Could you check a few things on this model? Use its own coordinates, in mm. A direction names the side the tool comes from. Coordinates: 2 decimals unless noted, no trailing zeros. Loops run counter-clockwise (first coordinate to the right, second up) from the corner with the lowest first, then second, coordinate; pieces in that order, holes last.
1) Imagine slicing it at A-A on z = 27.5. Please give me the cut outline in (x, y) (3 decimals).
2) Imagine slicing it at D-D on x = 36.5. Please give me the cut outline in (y, z), plus the area to 3 significant figures.
3) Imagine slicing it at C-C on z = 10. Please give me the cut outline in (x, y) (3 decimals), plus the area to 3 significant figures.
4) For faces 4 (the face through (67.07, -3, 11.686)), 5 (the face through (23.337, -4.217, 28.465)), 6 (the face through (36, -4, 26)), 7 (the face through (4.93, -5.15, 11.686)), which set-ups out of +Z, -Z, +X, -X, +Y, -Y let a thin tool reach every point of the face, with its end or its side?
5) If I drill on line 1 along Y through (x, z) = (50, 29); line 2 along X through (y, z) = (-3, 28.9); line 3 along Z through (x, y) = (66, -4), over which ranges is the centre line in solid material (lowest first)?
6) Will these pins go through, and if not, where does the flat tip stop? P1, Ø3.5, axis at y = -4.075, z = 10, coming from the +X side; P2, Ø1.5, axis at y = -6, z = 28.5, coming from the -X side; P3, Ø1.5, axis at y = -4, z = 21, coming from the +X side.
7) Thinking about a two-plate mould opening in Y: for faces 1 (the face through (62, -4, 10)), 2 (the face through (35, -8.15, 16)), 3 (the face through (57, -4, 31)), which applies, released by +Y, released by -Y, zero draft, split by the parting line, or undercut?
8) Imagine slicing it at B-B on y = -7.25. Please give me the cut outline in (x, z).
```python
from build123d import *

# Parameters (mm, degrees)
F1_DEPTH = 8.15
F3_D     = 4
F3_DEPTH = 5
F3_TIP   = 1.2017212381
F4_R     = 2
F5_DEPTH = 10
F6_R     = 2
F7_DEPTH = 10


with BuildPart() as f1:
    # F0 (on Front) → F1 (new body)
    with BuildSketch(Plane.XZ):
        Polygon((0, 20), (0, 0), (72, 0), (72, 20), (67.75, 31), (45.25, 31), (45.25, 26), (26.75, 26), (26.75, 31), (4.25, 31), align=None)
    extrude(amount=F1_DEPTH)

    # F3
    with Locations(Plane.XY.offset(31)):
        with Locations((21.75, -3), (50.25, -4.075)):
            Hole(F3_D / 2, depth=F3_DEPTH)
            with Locations((0, 0, -(F3_DEPTH + F3_TIP / 2))):  # 118° drill point
                Cone(0, F3_D / 2, F3_TIP, mode=Mode.SUBTRACT)

    # F4 (on face) → F5 (cut)
    with BuildSketch(Plane.YZ.offset(72)):
        with Locations((-4.075, 10)):
            Circle(F4_R)
    extrude(amount=-F5_DEPTH, mode=Mode.SUBTRACT)

    # F6 (on face) → F7 (cut)
    with BuildSketch(Plane(origin=(0, 0, 0), x_dir=(0, -1, 0), z_dir=(-1, 0, 0))):
        with Locations((4.075, 10)):
            Circle(F6_R)
    extrude(amount=-F7_DEPTH, mode=Mode.SUBTRACT)


solid = f1.part
```
Filled in:
1. outline: (2.898, -8.15) - (26.75, -8.15) - (26.75, 0) - (2.898, 0) - close; (45.25, -8.15) - (69.102, -8.15) - (69.102, 0) - (45.25, 0) - close; hole circle Ø4 at (21.75, -3); hole circle Ø4 at (50.25, -4.075)
2. outline: (-8.15, 0) - (0, 0) - (0, 26) - (-8.15, 26) - close
2. area: 212 mm2
3. outline: (0, -8.15) - (72, -8.15) - (72, -6.075) - (62, -6.075) - (62, -2.075) - (72, -2.075) - (72, 0) - (0, 0) - (0, -2.075) - (10, -2.075) - (10, -6.075) - (0, -6.075) - close
3. area: 507 mm2
4. face 4: +X
4. face 5: +Z
4. face 6: +Z, +Y, -Y
4. face 7: -X
5. line 1: y = -8.15 to -6.06, -2.09 to 0
5. line 2: x = 3.44 to 19.75, 23.75 to 26.75, 45.25 to 48.56, 51.94 to 68.56
5. line 3: z = 0 to 8, 12 to 31
6. P1: stops at x = 62
6. P2: stops at x = 2.99
6. P3: stops at x = 71.9
7. face 1: undercut
7. face 2: released by -Y
7. face 3: zero draft
8. outline: (0, 0) - (72, 0) - (72, 20) - (67.75, 31) - (45.25, 31) - (45.25, 26) - (26.75, 26) - (26.75, 31) - (4.25, 31) - (0, 20) - close
